Read the model definition and answer for the solid it produces. Units are mm, in the model's axes. A direction names the side the tool comes from. Give positions to 0.01 mm unless a question says otherwise; leave off trailing zeros. Write each loop counter-clockwise with the first axis right and the second up, starting at its lowest first coordinate (ties: lowest second). Pieces come first, ordered by that corner, then holes. Notation, with made-up numbers: (12.25, 59.25) - (49.25, 59.25) arc R30 ccw to (49.25, 86.25) - close; hole circle Ø5 at (33, 20.25). An arc over 180 degrees is marked (long way). Answer as CSV lines item,"result".
```python
from build123d import *

# Parameters (mm, degrees)
SKETCH2_R           = 64.77
BOSS_EXTRUDE1_DEPTH = 31.75
FILLET1_R           = 0.635
SKETCH3_R           = 29.21
CUT_EXTRUDE1_DEPTH  = 12.7
SKETCH4_R           = 9.525
CUT_EXTRUDE2_DEPTH  = 12.7
SKETCH5_R           = 7.62
CUT_EXTRUDE3_DEPTH  = 10.16


with BuildPart() as part:
    # Sketch2 → Boss-Extrude1 (new body)
    with BuildSketch(Plane(origin=(0, 0, 0), x_dir=(1, 0, 0), z_dir=(0, 1, 0))):
        with Locations(Location((0, 0, 0), (0, 0, 270))):
            Circle(SKETCH2_R)
    extrude(amount=BOSS_EXTRUDE1_DEPTH)

    # Fillet1
    fillet1_edges = [part.edges().sort_by_distance(p)[0] for p in [
        (0, 0, -64.77),
        (0, 31.75, -64.77),
    ]]
    fillet(fillet1_edges, radius=FILLET1_R)

    # Sketch3 → Cut-Extrude1 (cut)
    with BuildSketch(Plane(origin=(0, 31.75, 0), x_dir=(1, 0, 0), z_dir=(0, 1, 0))):
        with Locations(Location((0, 0, 0), (0, 0, 270))):
            Circle(SKETCH3_R)
    extrude(amount=-CUT_EXTRUDE1_DEPTH, mode=Mode.SUBTRACT)

    # Sketch4 → Cut-Extrude2 (cut)
    with BuildSketch(Plane(origin=(0, 19.05, 0), x_dir=(1, 0, 0), z_dir=(0, 1, 0))):
        with Locations(Location((0, 0, 0), (0, 0, 270))):
            Circle(SKETCH4_R)
    extrude(amount=-CUT_EXTRUDE2_DEPTH, mode=Mode.SUBTRACT)

    # Sketch5 → Cut-Extrude3 (cut)
    with BuildSketch(Plane(origin=(0, 31.75, 0), x_dir=(1, 0, 0), z_dir=(0, 1, 0))):
        with Locations(Location((0, -44.45, 0), (0, 0, 270))):
            Circle(SKETCH5_R)
        with Locations(Location((0, 44.45, 0), (0, 0, 90))):
            Circle(SKETCH5_R)
    extrude(amount=-CUT_EXTRUDE3_DEPTH, mode=Mode.SUBTRACT)


solid = part.part
```
(1) Find the intervals of material crossed by L1, parallel to Z at x = -3, y = 30.5; L2, parallel to X at y = 22, z = 0; L3, parallel to X at y = 22, z = -47, in increasing order.
Worked out:
L1,"z = -64.7 to -51.45, -37.45 to -29.06, 29.06 to 37.45, 51.45 to 64.7"
L2,"x = -64.77 to -29.21, 29.21 to 64.77"
L3,"x = -44.57 to -7.18, 7.18 to 44.57"
(2) A cutting plane is placed at C-C (y = 10.5). Write down the section's boundary in (x, z) (3 decimals).
Worked out:
outline,"circle Ø129.54 at (0, 0); hole circle Ø19.05 at (0, 0)"
(3) Each of these flat-tipped pins is pushed along its axis until it touches: P1, Ø5, axis at y = 21.5, z = -24.5, coming from the -X side; P2, Ø12, axis at x = 0, z = -44.45, coming from the +Y side; P3, Ø6, axis at x = 44, y = 14, coming from the -Z side. Where does it stop, or does it pass through?
Worked out:
P1,"stops at x = -60.92"
P2,"stops at y = 21.59"
P3,"stops at z = -50.14"
(4) A cutting plane is placed at A-A (z = 0). Write down the section's boundary in (x, y) (3 decimals).
Worked out:
outline,"(-64.77, 0.635) arc R0.635 ccw to (-64.135, 0) - (64.135, 0) arc R0.635 ccw to (64.77, 0.635) - (64.77, 31.115) arc R0.635 ccw to (64.135, 31.75) - (29.21, 31.75) - (29.21, 19.05) - (9.525, 19.05) - (9.525, 6.35) - (-9.525, 6.35) - (-9.525, 19.05) - (-29.21, 19.05) - (-29.21, 31.75) - (-64.135, 31.75) arc R0.635 ccw to (-64.77, 31.115) - close"
(5) A cutting plane is placed at B-B (x = 0). Write down the section's boundary in (y, z) (3 decimals), and give its area (3 significant figures).
Worked out:
outline,"(0, -64.135) arc R0.635 ccw to (0.635, -64.77) - (31.115, -64.77) arc R0.635 ccw to (31.75, -64.135) - (31.75, -52.07) - (21.59, -52.07) - (21.59, -36.83) - (31.75, -36.83) - (31.75, -29.21) - (19.05, -29.21) - (19.05, -9.525) - (6.35, -9.525) - (6.35, 9.525) - (19.05, 9.525) - (19.05, 29.21) - (31.75, 29.21) - (31.75, 36.83) - (21.59, 36.83) - (21.59, 52.07) - (31.75, 52.07) - (31.75, 64.135) arc R0.635 ccw to (31.115, 64.77) - (0.635, 64.77) arc R0.635 ccw to (0, 64.135) - close"
area,"2,820 mm^2"
(6) For faces 1 (the cylindrical face through (24.63, 25.49, 15.7)), 2 (the flat face through (1, 0, -1)), determine the directions among +Z, -Z, +X, -X, +Y, -Y from which every point of the face is accessible in a straight line to the end or side of a thin tool.
Worked out:
face 1,"+Y"
face 2,"+Z, -Z, +X, -X, -Y"
(7) The mould has two halves that part along Z. Classify faces 3 (the flat face through (-13, 31.75, 28)), 4 (the cylindrical face through (-0.335, 26.741, -36.837)), 5 (the cylindrical face through (-63.23, 15.66, -14.04)): +Z half, -Z half, draft (parallel to the pull), parting line (faces both ways), or undercut.
Worked out:
face 3,"draft"
face 4,"undercut"
face 5,"parting line"
